Input: dimensioned drawing with shaded views. Units: mm. Origin: part minimum x, y, z. A direction names the side the tool comes from. Round coordinates to 2 decimals unless told otherwise and drop trailing zeros. Order: outer loops, then holes, each group sorted by start corner. A loop starts at its lowest first (then second) coordinate and runs counter-clockwise, first axis right, second up.
Item 1: Mould query, pull axis Z, two halves, no side actions, for the marked faces 1, 2, 3 and 4. Classes: released by +Z, released by -Z, zero draft, split by the parting line, or undercut.
Item 2: Cut plane C-C on z = 30. Output: boundary loops of the cut face in (x, y), then the cut area to 3 significant figures.
Item 3: Cut plane B-B on y = 7. Output: boundary loops of the cut face in (x, z).
Item 4: First-contact query: pin 1 (5 mm diameter, centred on x = 31, z = 30, fed in from -Y). Flat tip, straight axial feed; report the tip coordinate or a pass-through.
Item 5: Cut plane D-D on y = 9.5. Output: boundary loops of the cut face in (x, z).
Item 6: Line query: L1, parallel to X at y = 9.25, z = 30; L2, parallel to X at y = 6, z = 51; L3, parallel to Z at x = 25, y = 7.5. Output: solid intervals per line, ascending.
Item 7: Reachability of the marked faces 5, 6 and 7 from +Z, -Z, +X, -X, +Y, -Y: full face, straight path, thin tool, end or side. Return the list, or none.
Item 8: Cut plane A-A on x = 16.5. Output: boundary loops of the cut face in (y, z).
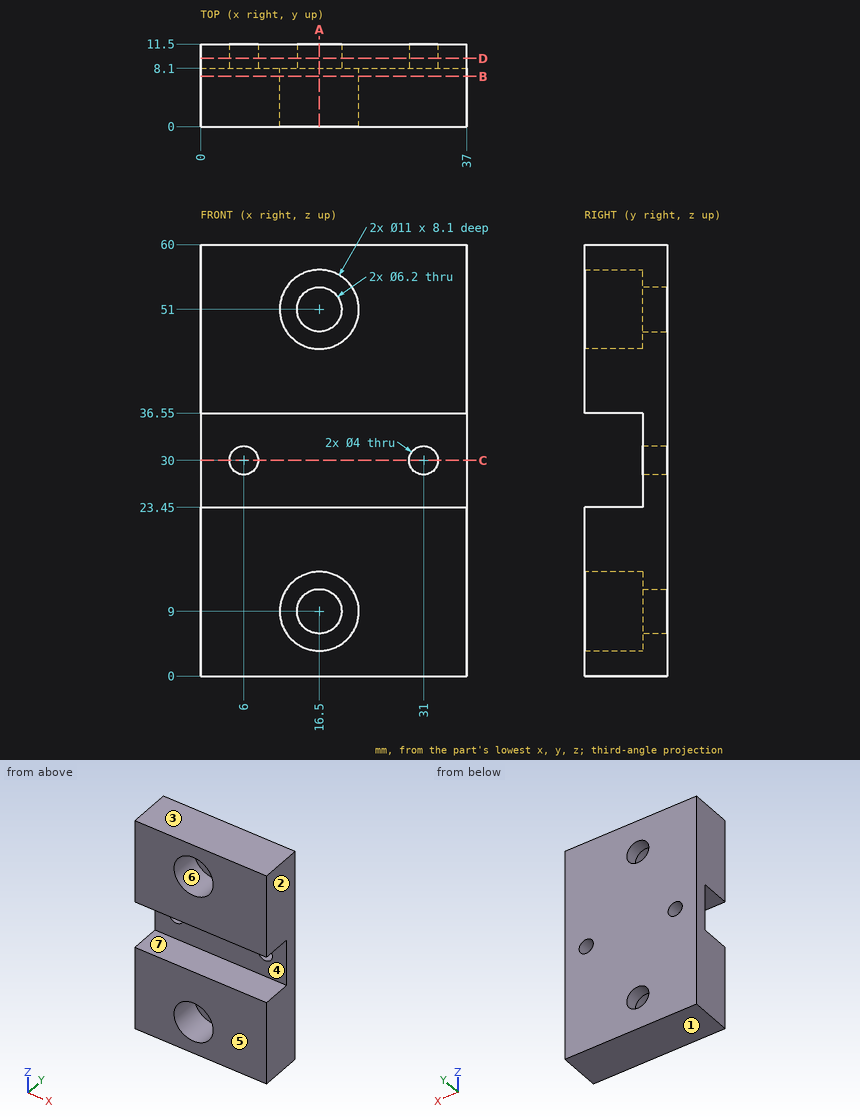
From the geometry:
1. face 1: released by -Z
1. face 2: zero draft
1. face 3: released by +Z
1. face 4: undercut
2. outline: (0, 8.1) - (4, 8.1) - (4, 11.5) - (0, 11.5) - close; (8, 8.1) - (29, 8.1) - (29, 11.5) - (8, 11.5) - close; (33, 8.1) - (37, 8.1) - (37, 11.5) - (33, 11.5) - close
2. area: 98.6 mm2
3. outline: (0, 0) - (37, 0) - (37, 23.45) - (0, 23.45) - close; (0, 36.55) - (37, 36.55) - (37, 60) - (0, 60) - close; hole circle Ø11 at (16.5, 9); hole circle Ø11 at (16.5, 51)
4. pin 1: stops at y = 8.1
5. outline: (0, 0) - (37, 0) - (37, 60) - (0, 60) - close; hole circle Ø4 at (6, 30); hole circle Ø6.2 at (16.5, 9); hole circle Ø6.2 at (16.5, 51); hole circle Ø4 at (31, 30)
6. L1: x = 0 to 4, 8 to 29, 33 to 37
6. L2: x = 0 to 11, 22 to 37
6. L3: z = 0 to 23.45, 36.55 to 60
7. face 5: +Z, -Z, +X, -X, -Y
7. face 6: -Y
7. face 7: +X, -X, -Y
8. outline: (0, 0) - (11.5, 0) - (11.5, 5.9) - (8.1, 5.9) - (8.1, 3.5) - (0, 3.5) - close; (0, 14.5) - (8.1, 14.5) - (8.1, 12.1) - (11.5, 12.1) - (11.5, 47.9) - (8.1, 47.9) - (8.1, 45.5) - (0, 45.5) - (0, 36.55) - (8.1, 36.55) - (8.1, 23.45) - (0, 23.45) - close; (0, 56.5) - (8.1, 56.5) - (8.1, 54.1) - (11.5, 54.1) - (11.5, 60) - (0, 60) - close
